```python
from build123d import *

# Parameters (mm, degrees)
SKETCH6_R          = 5.0419
CUT_EXTRUDE1_DEPTH = 44.553374001


with BuildPart() as part:
    # Sketch1 → Revolve1 (revolve)
    with BuildSketch(Plane(origin=(0, 0, 0), x_dir=(0, 0, -1), z_dir=(1, 0, 0))):
        Polygon((0, 0), (0, -5.08), (-30.58668, -5.08), (-30.58668, -3.81), (-28.68168, -3.81), (-28.68168, -1.27), (-30.58668, -1.27), (-30.58668, 0), align=None)
    revolve(axis=Axis((0, 0, 0), (0, -1, 0)))

    # Sketch6 → Cut-Extrude1 (cut, through all)
    with BuildSketch(Plane.XZ.offset(5.08)):
        with Locations(Location((0, 0, 0), (0, 0, 270))):
            Circle(SKETCH6_R)
    extrude(amount=-CUT_EXTRUDE1_DEPTH, mode=Mode.SUBTRACT)


solid = part.part
```
Geometry: final body of the model. Coordinates: model frame, mm. A direction names the side the tool comes from. Give positions to 0.01 mm unless a question says otherwise; leave off trailing zeros. Write each loop counter-clockwise with the first axis right and the second up, starting at its lowest first coordinate (ties: lowest second). Pieces come first, ordered by that corner, then holes.
1. Section query B-B, the plane x = 0. Return loops of the section in (y, z), then the cut area to 3 significant figures.
2. Pin query (flat end, axial travel): P1, Ø3, axis at x = 18.5, y = -3.5, coming from the -Z side; P2, Ø3, axis at x = 18, y = -2, coming from the -Z side; P3, Ø1.5, axis at x = 24.5, y = -3.5, coming from the +Z side. Return the tip coordinate at first contact, or that it passes through.
3. Draft query along Y for faces 3 (the flat face through (6, -5.08, 0)), 4 (the cylindrical face through (29.86, -4.44, -6.63)), 5 (the flat face through (-27.33, -3.81, -9.21)). Return one class per face: released by +Y, released by -Y, zero draft, split by the parting line, or undercut.
4. Section query D-D, the plane x = -21.5. Return loops of the section in (y, z), then the cut area to 3 significant figures.
5. Reachability of faces 1 (the cylindrical face through (10.985, -2.522, 26.495)), 2 (the cylindrical face through (29.86, -0.63, -6.63)) from +Z, -Z, +X, -X, +Y, -Y: full face, straight path, thin tool, end or side. Return the list, or none.
6. Section query C-C, the plane y = -2.45. Return loops of the section in (x, z).
7. Line query: probe 1 along X at (y, z) = (-1.9, 0); probe 2 along X at (y, z) = (-1.15, 0); probe 3 along Y at (x, z) = (13, 27.5). Output: solid intervals per line, ascending.
8. Section query A-A, the plane z = 0. Return loops of the section in (x, y), then the cut area to 3 significant figures.
Computed:
1. outline: (-5.08, -30.59) - (-3.81, -30.59) - (-3.81, -28.68) - (-1.27, -28.68) - (-1.27, -30.59) - (0, -30.59) - (0, -5.04) - (-5.08, -5.04) - close; (-5.08, 5.04) - (0, 5.04) - (0, 30.59) - (-1.27, 30.59) - (-1.27, 28.68) - (-3.81, 28.68) - (-3.81, 30.59) - (-5.08, 30.59) - close
1. area: 250 mm2
2. P1: stops at z = -25.41
2. P2: stops at z = -25.63
2. P3: stops at z = 19.19
3. face 3: released by -Y
3. face 4: zero draft
3. face 5: undercut
4. outline: (-5.08, -21.76) - (-3.81, -21.76) - (-3.81, -18.98) - (-1.27, -18.98) - (-1.27, -21.76) - (0, -21.76) - (0, 21.76) - (-1.27, 21.76) - (-1.27, 18.98) - (-3.81, 18.98) - (-3.81, 21.76) - (-5.08, 21.76) - close
4. area: 207 mm2
5. face 1: none
5. face 2: +Y, -Y
6. outline: circle Ø57.36 at (0, 0); hole circle Ø10.08 at (0, 0)
7. probe 1: x = -28.68 to -5.04, 5.04 to 28.68
7. probe 2: x = -30.59 to -5.04, 5.04 to 30.59
7. probe 3: y = -5.08 to -3.81, -1.27 to 0
8. outline: (-30.59, -5.08) - (-5.04, -5.08) - (-5.04, 0) - (-30.59, 0) - (-30.59, -1.27) - (-28.68, -1.27) - (-28.68, -3.81) - (-30.59, -3.81) - close; (5.04, -5.08) - (30.59, -5.08) - (30.59, -3.81) - (28.68, -3.81) - (28.68, -1.27) - (30.59, -1.27) - (30.59, 0) - (5.04, 0) - close
8. area: 250 mm2
